```python
from build123d import *

# Parameters (mm, degrees)
SKETCH_1_W               = 240
SKETCH_1_H               = 120
EXTRUDE_1_DEPTH          = 8
CUT_EXTRUDE_3_DEPTH      = 240
EXTRUDE_3_DEPTH          = 240
EXTRUDE_4_DEPTH          = 2
EXTRUDE_5_DEPTH          = 2
SKETCH_10_R              = 2
CUT_EXTRUDE_4_DEPTH      = 160.937906437
CUT_EXTRUDE_START        = -8
CUT_EXTRUDE_5_DEPTH      = 8
CUT_EXTRUDE_6_DEPTH      = 253.812214384
CUT_EXTRUDE_6_DEPTH_BACK = 253.812214384
CUT_EXTRUDE_7_DEPTH      = 255.695928005
EXTRUDE_6_DEPTH          = 240
CUT_EXTRUDE_8_REACH      = 254.456
SKETCH_19_W              = 5
SKETCH_19_H              = 131.995122826
EXTRUDE_7_DEPTH          = 8
CUT_EXTRUDE_9_DEPTH      = 25000
CUT_EXTRUDE_10_OUTLINE_R = 2.5
CUT_EXTRUDE_10_DEPTH     = 8
EXTRUDE_9_DEPTH          = 8
FILLET_1_R               = 20
EXTRUDE_11_DEPTH         = 250
SKETCH_26_W              = 10
SKETCH_26_H              = 15
EXTRUDE_12_DEPTH         = 0.1
CUT_EXTRUDE_11_DEPTH     = 280.220863782


# Read off the part's stored shape, not the designer's step: 切除-拉伸5, 切除-拉伸10
with BuildPart() as part:
    # 草图1 → 凸台-拉伸1 (new body)
    with BuildSketch(Plane.XY):
        with Locations((15.314885496, 17.910305344)):
            Rectangle(SKETCH_1_W, SKETCH_1_H)
    extrude(amount=EXTRUDE_1_DEPTH)

    # 草图5 → 切除-拉伸3 (cut)
    with BuildSketch(Plane.ZY.offset(104.685114504)):
        Polygon((0, -42.089694656), (8, -42.089694656), (1.137058799, -38.127373707), (0, -37.470892503), align=None)
    extrude(amount=-CUT_EXTRUDE_3_DEPTH, mode=Mode.SUBTRACT)

    # 草图6 → 凸台-拉伸3 (add)
    with BuildSketch(Plane.ZY.offset(104.685114504)):
        Polygon((8, -42.089694656), (34.641016151, -59.78029358), (8, -36.526716392), align=None)
    extrude(amount=-EXTRUDE_3_DEPTH)

    # 草图7 → 凸台-拉伸4 (add)
    with BuildSketch(Plane.ZY.offset(104.685114504)):
        Polygon((8, 10.562283697), (24.445035201, -50.880744528), (8, -36.526716392), align=None)
    extrude(amount=-EXTRUDE_4_DEPTH)

    # 草图8 → 凸台-拉伸5 (add)
    with BuildSketch(Plane(origin=(135.314885496, 0, 0), x_dir=(0, 0, -1), z_dir=(1, 0, 0))):
        Polygon((-8, 10.562283697), (-8, -36.526716392), (-24.445035201, -50.880744528), align=None)
    extrude(amount=-EXTRUDE_5_DEPTH)

    # 草图10 → 切除-拉伸4 (cut, through all)
    with BuildSketch(Plane(origin=(0, 0, 0), x_dir=(-1, 0, 0), z_dir=(0, 0, -1))):
        with Locations((-88.314885496, 72.410305344)):
            Circle(SKETCH_10_R)
        with Locations((-88.314885496, 42.410305344)):
            Circle(SKETCH_10_R)
        with Locations(Location((57.685114504, 42.410305344, 0), (0, 0, 180))):
            Circle(SKETCH_10_R)
        with Locations(Location((57.685114504, 72.410305344, 0), (0, 0, 180))):
            Circle(SKETCH_10_R)
        with Locations((97.685114504, 74.410305344)):
            Circle(SKETCH_10_R)
        with Locations((97.685114504, 50.410305344)):
            Circle(SKETCH_10_R)
        with Locations((71.685114504, 74.410305344)):
            Circle(SKETCH_10_R)
        with Locations((71.685114504, 50.410305344)):
            Circle(SKETCH_10_R)
        with Locations(Location((-102.314885496, 50.410305344, 0), (0, 0, 180))):
            Circle(SKETCH_10_R)
        with Locations(Location((-128.314885496, 50.410305344, 0), (0, 0, 180))):
            Circle(SKETCH_10_R)
        with Locations(Location((-128.314885496, 74.410305344, 0), (0, 0, 180))):
            Circle(SKETCH_10_R)
        with Locations(Location((-102.314885496, 74.410305344, 0), (0, 0, 180))):
            Circle(SKETCH_10_R)
    extrude(amount=-CUT_EXTRUDE_4_DEPTH, mode=Mode.SUBTRACT)

    # 切除-拉伸5 outline → 切除-拉伸5 (cut)
    with BuildSketch(Plane.XY.offset(8).offset(CUT_EXTRUDE_START)):
        with BuildLine():
            Line((-85.305572399, 41.762915626), (-54.149293781, -12.223394737))
            add(Edge.make_bspline(
                [(-54.149293781, -12.223394737), (-42.947902037, -24.544925656), (-30.906405911, -28.185377973), (-18.024805405, -30.145621528), (17.539613385, -54.788683367), (6.898291227, -20.904473339), (10.818778338, -6.902733658), (10.818778338, 6.538936436), (-9.063692009, 20.540676117)],
                knots=[0, 0, 0, 0, 0, 0, 0, 0, 0, 1, 1, 1, 1, 1, 1, 1, 1, 1], degree=8))
            Line((-9.063692009, 20.540676117), (-84.150317121, 43.220048807))
            ThreePointArc((-84.150317121, 43.220048807), (-85.223061497, 42.884024389), (-85.305572399, 41.762915626))
        make_face()
        with BuildLine():
            Line((114.780088113, 43.220048807), (39.693463001, 20.540676117))
            add(Edge.make_bspline(
                [(39.693463001, 20.540676117), (19.810992654, 6.538936436), (19.810992654, -6.902733658), (23.731479765, -20.904473339), (13.090157607, -54.788683367), (48.654576397, -30.145621528), (61.536176903, -28.185377973), (73.577673029, -24.544925656), (84.779064774, -12.223394737)],
                knots=[0, 0, 0, 0, 0, 0, 0, 0, 0, 1, 1, 1, 1, 1, 1, 1, 1, 1], degree=8))
            Line((84.779064774, -12.223394737), (115.935343391, 41.762915626))
            ThreePointArc((115.935343391, 41.762915626), (115.85283249, 42.884024389), (114.780088113, 43.220048807))
        make_face()
        with BuildLine():
            Line((73.645432244, 77.910305344), (-43.015661252, 77.910305344))
            ThreePointArc((-43.015661252, 77.910305344), (15.314885496, 50.054205438), (73.645432244, 77.910305344))
        make_face()
    extrude(amount=CUT_EXTRUDE_5_DEPTH, mode=Mode.SUBTRACT)

    # 草图14 → 切除-拉伸6 (cut, two sides: drawn at the far end of the back side and taken through both)
    with BuildSketch(Plane(origin=(-102.685114504, 0, 0), x_dir=(0, 0, -1), z_dir=(1, 0, 0)).offset(-CUT_EXTRUDE_6_DEPTH_BACK)):
        Polygon((-8, -36.526716392), (-8, 10.562283697), (-24.445035201, -50.880744528), align=None)
    extrude(amount=CUT_EXTRUDE_6_DEPTH + CUT_EXTRUDE_6_DEPTH_BACK, mode=Mode.SUBTRACT)

    # 草图15 → 切除-拉伸7 (cut, through all)
    with BuildSketch(Plane(origin=(135.314885496, 0, 0), x_dir=(0, 0, -1), z_dir=(1, 0, 0))):
        Polygon((-8, -36.526716392), (-8, -49.78029358), (-41.869464541, -71.644239127), (-41.869464541, -31.236191865), align=None)
    extrude(amount=-CUT_EXTRUDE_7_DEPTH, mode=Mode.SUBTRACT)

    # 草图17 → 凸台-拉伸6 (add)
    with BuildSketch(Plane.ZY.offset(104.685114504)):
        Polygon((8, -42.089694656), (0, -37.470892503), (0, -57.621161091), (8, -62.239963244), align=None)
    extrude(amount=-EXTRUDE_6_DEPTH)

    # 草图18 → 切除-拉伸8 (cut, up to next)
    with BuildSketch(Plane.ZY.offset(104.685114504), mode=Mode.PRIVATE) as cut_extrude_8_sk1:
        Polygon((8, -54.084817482), (0, -47.372020433), (0, -57.621161091), (8, -62.239963244), align=None)
    cut_extrude_8_tool1 = extrude(cut_extrude_8_sk1.sketch, amount=-CUT_EXTRUDE_8_REACH, mode=Mode.PRIVATE) & part.part
    add(cut_extrude_8_tool1.solids().sort_by_distance((-104.685115, -55.22205, 3.848297))[0], mode=Mode.SUBTRACT)

    # 草图19 → 凸台-拉伸7 (add)
    with BuildSketch(Plane.XY):
        with Locations((-107.185114504, 11.912743931)):
            Rectangle(SKETCH_19_W, SKETCH_19_H)
        with Locations((137.814885496, 11.912743931)):
            Rectangle(SKETCH_19_W, SKETCH_19_H)
    extrude(amount=EXTRUDE_7_DEPTH)

    # 草图20 → 切除-拉伸9 (cut, symmetric)
    with BuildSketch(Plane(origin=(-104.685114504, 0, 0), x_dir=(0, 0, -1), z_dir=(1, 0, 0))):
        Polygon((0, -47.372020433), (-8, -54.084817482), (0, -54.084817482), align=None)
    extrude(amount=CUT_EXTRUDE_9_DEPTH, both=True, mode=Mode.SUBTRACT)

    # 切除-拉伸10 outline → 切除-拉伸10 (cut)
    with BuildSketch(Plane.XY.offset(8).offset(CUT_EXTRUDE_START)):
        with BuildLine():
            Line((140.314885496, -45.465697905), (140.314885496, 50.054205438))
            add(Edge.make_bspline(
                [(140.314885496, 50.054205438), (137.158486233, 30.091614758), (88.199951512, 16.126556544), (112.176664555, -11.734503746), (106.252853678, -38.244537039), (137.741665906, -24.260832479), (140.314885496, -45.465697905)],
                knots=[0, 0, 0, 0, 0, 0, 0, 1, 1, 1, 1, 1, 1, 1], degree=6))
        make_face()
        with BuildLine():
            Line((-109.685114504, 50.054205438), (-109.685114504, -45.465697905))
            add(Edge.make_bspline(
                [(-109.685114504, -45.465697905), (-107.111894913, -24.260832479), (-75.623082686, -38.244537039), (-81.546893563, -11.734503746), (-57.57018052, 16.126556544), (-106.528715241, 30.091614758), (-109.685114504, 50.054205438)],
                knots=[0, 0, 0, 0, 0, 0, 0, 1, 1, 1, 1, 1, 1, 1], degree=6))
        make_face()
        with Locations((8.984830356, -36.133723352)):
            Circle(CUT_EXTRUDE_10_OUTLINE_R)
        with Locations((21.644940637, -36.133723352)):
            Circle(CUT_EXTRUDE_10_OUTLINE_R)
    extrude(amount=CUT_EXTRUDE_10_DEPTH, mode=Mode.SUBTRACT)

    # 草图23 → 凸台-拉伸9 (add)
    with BuildSketch(Plane.XY.offset(8)):
        with BuildLine():
            Line((-109.685114504, 77.910305344), (-43.015661252, 77.910305344))
            Line((-43.015661252, 77.910305344), (-110.286718721, 104.141059297))
            ThreePointArc((-110.286718721, 104.141059297), (-116.285944727, 103.178230136), (-118.368287428, 97.470200569))
            Line((-118.368287428, 97.470200569), (-109.685114504, 50.054205438))
            Line((-109.685114504, 50.054205438), (-109.685114504, 77.910305344))
        make_face()
        with BuildLine():
            Line((148.998058421, 97.470200569), (140.314885496, 50.054205438))
            Line((140.314885496, 50.054205438), (140.314885496, 77.910305344))
            Line((140.314885496, 77.910305344), (73.645432244, 77.910305344))
            Line((73.645432244, 77.910305344), (140.916489713, 104.141059297))
            ThreePointArc((140.916489713, 104.141059297), (146.915715719, 103.178230136), (148.998058421, 97.470200569))
        make_face()
    extrude(amount=-EXTRUDE_9_DEPTH)

    # 圆角1
    fillet_1_edges = [part.edges().sort_by_distance(p)[0] for p in [
        (73.645432244, 77.910305344, 4),
        (-43.015661252, 77.910305344, 4),
    ]]
    fillet(fillet_1_edges, radius=FILLET_1_R)

    # 草图25 → 凸台-拉伸11 (add)
    with BuildSketch(Plane.ZY.offset(109.685114504)):
        Polygon((0, -47.372020433), (8, -54.084817482), (8, -59.084817482), (0, -52.372020433), align=None)
    extrude(amount=-EXTRUDE_11_DEPTH)

    # 草图26 → 凸台-拉伸12 (add)
    with BuildSketch(Plane.XY.offset(8)):
        with Locations((-94.685114504, -51.584817482)):
            Rectangle(SKETCH_26_W, SKETCH_26_H)
        with Locations((-74.685114504, -51.584817482)):
            Rectangle(SKETCH_26_W, SKETCH_26_H)
        with Locations((-54.685114504, -51.584817482)):
            Rectangle(SKETCH_26_W, SKETCH_26_H)
        with Locations((-34.685114504, -51.584817482)):
            Rectangle(SKETCH_26_W, SKETCH_26_H)
        with Locations((-14.685114504, -51.584817482)):
            Rectangle(SKETCH_26_W, SKETCH_26_H)
        with Locations((5.314885496, -51.584817482)):
            Rectangle(SKETCH_26_W, SKETCH_26_H)
        with Locations((25.314885496, -51.584817482)):
            Rectangle(SKETCH_26_W, SKETCH_26_H)
        with Locations((45.314885496, -51.584817482)):
            Rectangle(SKETCH_26_W, SKETCH_26_H)
        with Locations((65.314885496, -51.584817482)):
            Rectangle(SKETCH_26_W, SKETCH_26_H)
        with Locations((85.314885496, -51.584817482)):
            Rectangle(SKETCH_26_W, SKETCH_26_H)
        with Locations((105.314885496, -51.584817482)):
            Rectangle(SKETCH_26_W, SKETCH_26_H)
        with Locations((125.314885496, -51.584817482)):
            Rectangle(SKETCH_26_W, SKETCH_26_H)
    extrude(amount=EXTRUDE_12_DEPTH)

    # 草图27 → 切除-拉伸11 (cut, through all)
    with BuildSketch(Plane.ZY.offset(109.685114504)):
        Polygon((8, -54.182166182), (0, -47.372020433), (0, -52.372020433), (8, -59.084817482), (8.781870659, -59.891234403), (8.781870659, -54.740884863), align=None)
    extrude(amount=-CUT_EXTRUDE_11_DEPTH, mode=Mode.SUBTRACT)


solid = part.part
```
Geometry check sheet. Reference: the model listing, model coordinates, mm. A direction names the side the tool comes from. Coordinates: 2 decimals unless noted, no trailing zeros. Write each loop counter-clockwise with the first axis right and the second up, starting at its lowest first coordinate (ties: lowest second). Pieces come first, ordered by that corner, then holes. Notation, with made-up numbers: (79.25, 4.5) -> (98.25, 4.5) arc R27 cw to (98.25, 42.5) -> close; hole circle Ø6 at (-15.5, 39). An arc over 180 degrees is marked (long way). Use CSV: the item, a comma, the result in double quotes. Start each with the question number.
Item 1: Cross-section at C-C, the plane z = 6. State how many separate pieces and enclosed holes the cut face has, plus the area to 3 significant figures.
Item 2: Mould release check, pull along X, two halves, no side actions. Record for faces 6 (the flat face through (144.717, 74.094, 4.056)), 7 (the cylindrical face through (8.443, -38.574, 3.944)), 8 (the flat face through (65, -49, 8.1)): released by +X, released by -X, zero draft, split by the parting line, or undercut.
Item 3: Depth check by flat-ended pin: pin 1 Ø8 at (x, y) = (8.98, -36.13) entering from +Z; pin 2 Ø2 at (y, z) = (25, 6.5) entering from -X; pin 3 Ø1.5 at (y, z) = (53.5, 7) entering from +X; pin 4 Ø3 at (x, y) = (-57.69, 72.41) entering from -Z. Enter the tip coordinate at first touch or a pass-through.
Item 4: Thickness scan on line 1 (X direction, y = 50, z = 6.75); line 2 (X direction, y = -38, z = 7); line 3 (Y direction, x = 126.5, z = 3.5). Record the ranges inside material, lowest first.
Item 5: Set-up check for faces 1 (the flat face through (13.565, -50.825, 4.056)), 2 (the flat face through (-75, -49, 8.1)), 3 (the flat face through (-69.946, 15.148, 3.944)), 4 (the flat face through (140.315, -49, 5)), 5 (the cylindrical face through (-43.65, 77.61, 4.06)): record each of +Z, -Z, +X, -X, +Y, -Y from which the full face is reachable in a straight line by a thin tool's end or side.
Item 6: Cross-section at A-A, the plane y = 65. Record the cut outline in (x, z).
Item 7: Cross-section at B-B, the plane x = -67. Record the cut outline in (y, z).
Answers:
1,separate pieces,"1"
1,enclosed holes,"16"
1,area,"21,400 mm^2"
2,face 6,"released by +X"
2,face 7,"undercut"
2,face 8,"zero draft"
3,pin 1,"z = 8"
3,pin 2,"x = -91.7"
3,pin 3,"x = 141.08"
3,pin 4,"through"
4,line 1,"-109.68 to -99.64, -95.73 to -73.64, -69.73 to 100.36, 104.27 to 126.36, 130.27 to 140.31"
4,line 2,"-106.32 to 7.32, 10.65 to 19.98, 23.31 to 136.94"
4,line 3,"-50.35 to -30.71, 30.82 to 49.57, 51.25 to 73.57, 75.25 to 98.52"
5,face 1,"-Z, +X, -X, -Y"
5,face 2,"+Z, +X, -X, +Y, -Y"
5,face 3,"+Z, -Z"
5,face 4,"+Z, -Z, +X, -Y"
5,face 5,"+Z, -Z, +Y"
6,outline,"(-112.42, 0) -> (-29.61, 0) -> (-29.61, 8) -> (-112.42, 8) -> close; (60.24, 0) -> (143.05, 0) -> (143.05, 8) -> (60.24, 8) -> close"
7,outline,"(-54.18, 8) -> (-47.37, 0) -> (10.04, 0) -> (10.04, 8) -> close; (38.04, 0) -> (87.26, 0) -> (87.26, 8) -> (38.04, 8) -> close"
